from build123d import *

# Parameters (mm, degrees)
SCHIZZO1_W                     = 50
SCHIZZO1_H                     = 3
ESTRUSIONE_ESTRUSIONE1_DEPTH   = 20
ESTRUSIONE_ESTRUSIONE2_DEPTH   = 20
ESTRUSIONE_ESTRUSIONE2_2_DEPTH = 20
RACCORDO2_R                    = 6
RACCORDO3_DEPTH                = 20
RACCORDO4_R                    = 6
RACCORDO5_R                    = 6
RACCORDO7_R                    = 2
RACCORDO8_R                    = 2
SCHIZZO5_W                     = 11.5
SCHIZZO5_H                     = 20
TAGLIO_ESTRUSIONE2_DEPTH       = 3
ESTRUSIONE_ESTRUSIONE7_DEPTH   = 20
SCHIZZO12_R                    = 1.15
ESTRUSIONE_ESTRUSIONE9_DEPTH   = 3
TAGLIO_ESTRUSIONE4_DEPTH       = 52.461506674
TAGLIO_ESTRUSIONE4_DEPTH_BACK  = 52.461506674


with BuildPart() as part:
    # Schizzo1 → Estrusione-Estrusione1 (new body)
    with BuildSketch(Plane.XY):
        with Locations((25, 1.5)):
            Rectangle(SCHIZZO1_W, SCHIZZO1_H)
    extrude(amount=ESTRUSIONE_ESTRUSIONE1_DEPTH)

    # Schizzo5 → Taglio-Estrusione2 (cut)
    with BuildSketch(Plane(origin=(0, 3, 0), x_dir=(1, 0, 0), z_dir=(0, 1, 0))):
        with Locations((5.75, -10)):
            Rectangle(SCHIZZO5_W, SCHIZZO5_H)
        with Locations((44.25, -10)):
            Rectangle(SCHIZZO5_W, SCHIZZO5_H)
    extrude(amount=-TAGLIO_ESTRUSIONE2_DEPTH, mode=Mode.SUBTRACT)



with BuildPart() as body_2:
    # Schizzo2 → Estrusione-Estrusione2 (new body)
    with BuildSketch(Plane.XY.offset(20)):
        Polygon((12, 3), (21.667680152, 19.610006491), (21.667680152, 25.610006491), (18.742038116, 30.677367142), (23.742038116, 30.677367142), (24.8, 24.677367142), (23.500961894, 23.927367142), (24.8, 22.837344747), (24.8, 19.837344747), (15, 3), align=None)
    extrude(amount=-ESTRUSIONE_ESTRUSIONE2_DEPTH)

    # Raccordo2
    # the kernel refuses this fillet: 6 mm, written as the material it takes off along each edge
    with BuildSketch(Plane(origin=(23.742038116, 30.677367142, 32.586494468), x_dir=(-1, 0, 0), z_dir=(0, 0, -1))) as raccordo2_piece_1:
        with BuildLine():
            CenterArc((RACCORDO2_R * 0.839099631177, -RACCORDO2_R), RACCORDO2_R, 90, 80)
            Line((-RACCORDO2_R * 0.145708121835, -RACCORDO2_R * 0.826351822333), (0, 0))
            Line((0, 0), (RACCORDO2_R * 0.839099631177, 0))
        make_face()
    extrude(amount=45.172988935, mode=Mode.SUBTRACT)

    # Raccordo5
    raccordo5_edges = [body_2.edges().sort_by_distance(p)[0] for p in [
        (21.667680152, 19.610006491, 10),
    ]]
    fillet(raccordo5_edges, radius=RACCORDO5_R)

    # Raccordo8
    raccordo8_edges = [body_2.edges().sort_by_distance(p)[0] for p in [
        (15, 3, 10),
    ]]
    fillet(raccordo8_edges, radius=RACCORDO8_R)

    # Schizzo9 → Estrusione-Estrusione7 (add)
    with BuildSketch(Plane.XY.offset(20)):
        Polygon((24.564100135, 19.432046037), (22.884294771, 16.545978484), (26.884294771, 16.545978484), (25.204489408, 19.432046037), align=None)
    extrude(amount=-ESTRUSIONE_ESTRUSIONE7_DEPTH)


with BuildPart() as body_3:
    # Schizzo2 → Estrusione-Estrusione2 2 (new body)
    with BuildSketch(Plane.XY.offset(20)):
        Polygon((26.499038106, 23.927367142), (25.2, 22.837344747), (25.2, 19.837344747), (35, 3), (38, 3), (28.332319848, 19.610006491), (28.332319848, 25.610006491), (31.257961884, 30.677367142), (26.257961884, 30.677367142), (25.2, 24.677367142), align=None)
    extrude(amount=-ESTRUSIONE_ESTRUSIONE2_2_DEPTH)

    # Raccordo3: read off the stored shape, not the designer's step
    # Raccordo3 outline → Raccordo3 (cut)
    with BuildSketch(Plane.XY):
        with BuildLine():
            add(Edge.make_bspline(
                [(31.257961884, 30.677367142), (26.252870263, 30.648491125), (25.38373076, 25.719356061)],
                knots=[0, 0, 0, 1, 1, 1], degree=2, weights=[1, 0.767895459, 1]))
            Line((31.257961884, 30.677367142), (26.257961884, 30.677367142))
            Line((26.257961884, 30.677367142), (25.38373076, 25.719356061))
        make_face()
    extrude(amount=RACCORDO3_DEPTH, mode=Mode.SUBTRACT)

    # Raccordo4
    raccordo4_edges = [body_3.edges().sort_by_distance(p)[0] for p in [
        (28.332319848, 19.610006491, 10),
    ]]
    fillet(raccordo4_edges, radius=RACCORDO4_R)

    # Raccordo7
    raccordo7_edges = [body_3.edges().sort_by_distance(p)[0] for p in [
        (35, 3, 10),
    ]]
    fillet(raccordo7_edges, radius=RACCORDO7_R)


with BuildPart() as part_1:
    add(part.part)

    add(body_2.part)  # Estrusione-Estrusione9 merges body 2

    add(body_3.part)  # Estrusione-Estrusione9 merges body 3
    # Schizzo12 → Estrusione-Estrusione9 (add)
    with BuildSketch(Plane(origin=(0, 3, 0), x_dir=(1, 0, 0), z_dir=(0, 1, 0))):
        Polygon((11.5, 0), (38.5, 0), (38.5, 7), (29, 7), (21, 7), (11.5, 7), align=None)
        with Locations(Location((16.5, 4, 0), (0, 0, 270))):
            Circle(SCHIZZO12_R, mode=Mode.SUBTRACT)
        with Locations(Location((33.5, 4, 0), (0, 0, 270))):
            Circle(SCHIZZO12_R, mode=Mode.SUBTRACT)
    extrude(amount=-ESTRUSIONE_ESTRUSIONE9_DEPTH)

    # Schizzo13 → Taglio-Estrusione4 (cut, two sides: drawn at the far end of the back side and taken through both)
    with BuildSketch(Plane(origin=(0, 3, 0), x_dir=(1, 0, 0), z_dir=(0, 1, 0)).offset(-TAGLIO_ESTRUSIONE4_DEPTH_BACK)):
        with BuildLine():
            Line((21, 7), (21, 4.031977604))
            ThreePointArc((21, 4.031977604), (25, 0.031977604), (29, 4.031977604))
            Line((29, 4.031977604), (29, 7))
            Line((29, 7), (21, 7))
        make_face()
    extrude(amount=TAGLIO_ESTRUSIONE4_DEPTH + TAGLIO_ESTRUSIONE4_DEPTH_BACK, mode=Mode.SUBTRACT)


solid = part_1.part
Can you work these out from the model? Positions are in its coordinate system, mm. A direction names the side the tool comes from. Coordinates: 2 decimals unless noted, no trailing zeros. Loops run counter-clockwise (first coordinate to the right, second up) from the corner with the lowest first, then second, coordinate; pieces in that order, holes last. Notation, with made-up numbers: M 79.5,46.5 L 83.5,46.5 A11 ccw 83.5,56.5 Z; hole C 8.5,25.5 d3. An arc over 180 degrees is marked long. Return JSON: item names as keys, results as strings. Group by question number.
Item 1: Imagine slicing it at A-A (y = 3.5). Please give me the cut outline in (x, z).
Item 2: Imagine slicing it at B-B (x = 20). Please give me the cut outline in (y, z).
Item 3: Thinking about a two-plate mould opening in X: for faces 1 (the cylindrical face through (15.377, 1.521, -4.249)), 2 (the flat face through (24.8, 21, 10)), 3 (the cylindrical face through (21.455, 19.645, 9.86)), 4 (the flat face through (33.635, 10.499, 10.14)), which applies, released by +X, released by -X, zero draft, split by the parting line, or undercut?
Item 4: Imagine slicing it at C-C (x = 16.5). Please give me the cut outline in (y, z), and give its area (3 significant figures).
Item 5: If I drill on L1, parallel to X at y = 2.3, z = -4; L2, parallel to X at y = 23, z = 1.75; L3, parallel to Y at x = 31, z = 12.5, over which ranges is the centre line in solid material (lowest first)? Write a range as from..to.
Item 6: I'm going to push flat-ended pins straight in: pin 1 Ø1.5 at (y, z) = (9.5, 4) entering from +X; pin 2 Ø1.3 at (y, z) = (23.5, 14) entering from +X; pin 3 Ø3 at (x, z) = (16.5, -4) entering from +Y. Where does each tip first touch, or does it pass through?
Item 7: On a 3-axis mill with a long thin cutter (end or side, diameter ignored), from which of +Z, -Z, +X, -X, +Y, -Y can I reach the whole of each face in a straight line? I mean faces 5 (the flat face through (28.332, 23, 10)), 6 (the flat face through (25.293, 25.206, 10.14)), 7 (the flat face through (19.283, 10.358, 10.14)), 8 (the flat face through (16.365, 10.499, 10.14)), 9 (the flat face through (29.7, 16.9, 0)). Say none if no direction works.
Verdict:
{
 "1": {"outline": "M 12.29,0 L 15.17,0 L 15.17,20 L 12.29,20 Z; M 34.83,0 L 37.71,0 L 37.71,20 L 34.83,20 Z"},
 "2": {"outline": "M 0,-7 L 3,-7 L 3,20 L 0,20 Z; M 11.59,0 L 16.74,0 L 16.74,20 L 11.59,20 Z; M 28.5,0 L 30.54,0 L 30.54,20 L 28.5,20 Z"},
 "3": {"face 1": "undercut", "face 2": "undercut", "face 3": "released by -X", "face 4": "released by +X"},
 "4": {"outline": "M 0,-7 L 3,-7 L 3,-5.15 L 0,-5.15 Z; M 0,-2.85 L 3,-2.85 L 3,20 L 0,20 Z; M 5.58,0 L 10.73,0 L 10.73,20 L 5.58,20 Z", "area": "177 mm^2"},
 "5": {"L1": "x = 11.5..15.35, 17.65..21, 29..32.35, 34.65..38.5", "L2": "x = 21.67..24.61, 25.39..28.33", "L3": "y = 0..3, 9.87..15.03, 30.23..30.67"},
 "6": {"pin 1": "stops at x = 34.65", "pin 2": "stops at x = 28.33", "pin 3": "stops at y = 3"},
 "7": {"face 5": "+Z, -Z, +X", "face 6": "+Z, -Z, +Y", "face 7": "+Z, -Z", "face 8": "+Z, -Z, -X", "face 9": "-Z, +X, -X, +Y"}
}
